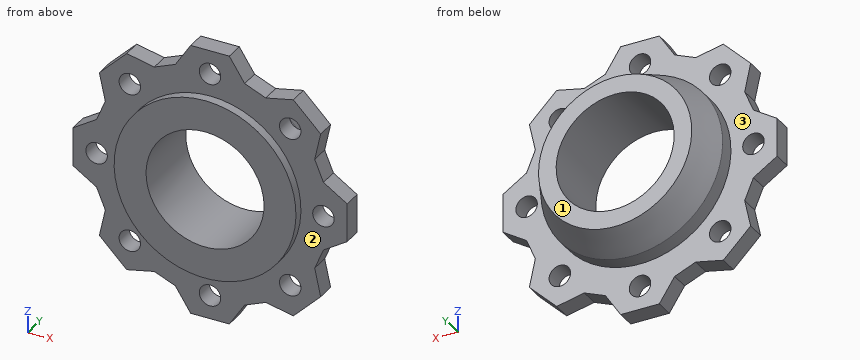
```python
from build123d import *

# Parameters (mm, degrees)
SKETCH2_R           = 3.5
SKETCH2_R_2         = 19.25
BOSS_EXTRUDE1_DEPTH = 6


with BuildPart() as part:
    # Sketch2 → Boss-Extrude1 (new body)
    with BuildSketch(Plane(origin=(0, 0, 0), x_dir=(1, 0, 0), z_dir=(0, 1, 0))):
        Polygon((27.188255737, 36.09780118), (18.172644276, 34.153257531), (11.3, 37), (6.3, 44.75), (-6.3, 44.75), (-11.3, 37), (-18.172644276, 34.153257531), (-27.188255737, 36.09780118), (-36.09780118, 27.188255737), (-34.153257531, 18.172644276), (-37, 11.3), (-44.75, 6.3), (-44.75, -6.3), (-37, -11.3), (-34.153257531, -18.172644276), (-36.09780118, -27.188255737), (-27.188255737, -36.09780118), (-18.172644276, -34.153257531), (-11.3, -37), (-6.3, -44.75), (6.3, -44.75), (11.3, -37), (18.172644276, -34.153257531), (27.188255737, -36.09780118), (36.09780118, -27.188255737), (34.153257531, -18.172644276), (37, -11.3), (44.75, -6.3), (44.75, 6.3), (37, 11.3), (34.153257531, 18.172644276), (36.09780118, 27.188255737), align=None)
        with Locations(Location((0, 37, 0), (0, 0, 270))):
            Circle(SKETCH2_R, mode=Mode.SUBTRACT)
        with Locations(Location((26.162950904, 26.162950904, 0), (0, 0, 270))):
            Circle(SKETCH2_R, mode=Mode.SUBTRACT)
        with Locations(Location((37, 0, 0), (0, 0, 270))):
            Circle(SKETCH2_R, mode=Mode.SUBTRACT)
        with Locations(Location((26.162950904, -26.162950904, 0), (0, 0, 270))):
            Circle(SKETCH2_R, mode=Mode.SUBTRACT)
        with Locations(Location((0, -37, 0), (0, 0, 270))):
            Circle(SKETCH2_R, mode=Mode.SUBTRACT)
        with Locations(Location((-26.162950904, -26.162950904, 0), (0, 0, 270))):
            Circle(SKETCH2_R, mode=Mode.SUBTRACT)
        with Locations(Location((-37, 0, 0), (0, 0, 270))):
            Circle(SKETCH2_R, mode=Mode.SUBTRACT)
        with Locations(Location((-26.162950904, 26.162950904, 0), (0, 0, 270))):
            Circle(SKETCH2_R, mode=Mode.SUBTRACT)
        with Locations(Location((0, 0, 0), (0, 0, 270))):
            Circle(SKETCH2_R_2, mode=Mode.SUBTRACT)
    extrude(amount=BOSS_EXTRUDE1_DEPTH)

    # Sketch3 → Revolve1 (revolve)
    with BuildSketch(Plane.XY, mode=Mode.PRIVATE) as revolve1_sk:
        Polygon((-19.25, 21), (-25, 21), (-29.663076582, 11), (-29.663076582, -3), (-19.25, -3), align=None)
    revolve(revolve1_sk.sketch.rotate(Axis((0, 33.758219329, 0), (0, -1, 0)), 270), axis=Axis((0, 33.758219329, 0), (0, -1, 0)))


solid = part.part
```
CAD build for the part. Positions are in the model's coordinates, mm. Face numbers are marked on the shaded views. A direction names the side the tool comes from. Round coordinates to 2 decimals unless told otherwise and drop trailing zeros. Loops run counter-clockwise (first coordinate to the right, second up) from the corner with the lowest first, then second, coordinate; pieces in that order, holes last. Notation, with made-up numbers: M 65.5,54 L 106.5,54 A11 cw 106.5,61 Z; hole C -34.5,-24 d11. An arc over 180 degrees is marked long. Return JSON: item names as keys, results as strings. Group by question number.
(1) Drop flat-ended pins along their axis: P1, Ø8, axis at x = -34.5, y = 8, coming from the -Z side; P2, Ø9, axis at x = 0, z = -37, coming from the -Y side; P3, Ø10, axis at y = 3.5, z = -12.5, coming from the -X side; P4, Ø8, axis at x = -33, y = 15, coming from the -Z side. Give the stop position or say it passes through.
(2) Saw through at A-A, the plane x = 0. List the corners of the cut face in (y, z).
(3) Wall check: probe 1 along X at (y, z) = (3.25, 0); probe 2 along X at (y, z) = (11, 0); probe 3 along Y at (x, z) = (-2, -34). Give the ranges that are in metal, low to high. Write a range as [from, to].
(4) Saw through at C-C, the plane x = -38.5. List the corners of the cut face in (y, z), and give its area (3 significant figures).
(5) Saw through at B-B, the plane z = 0. List the corners of the cut face in (x, y).
(6) Tool access for the marked faces 1, 2 and 3: list every direction of +Z, -Z, +X, -X, +Y, -Y with a clear straight run to the whole face (end or side of a thin tool).
(7) Saw through at D-D, the plane y = 16.75. List the corners of the cut face in (x, z).
Answer list:
{
 "1": {"P1": "z = -32.25", "P2": "y = 0", "P3": "x = -42.89", "P4": "through"},
 "2": {"outline": "M -3,-29.66 L 0,-29.66 L 0,-33.5 L 6,-33.5 L 6,-29.66 L 11,-29.66 L 21,-25 L 21,-19.25 L -3,-19.25 Z; M -3,19.25 L 21,19.25 L 21,25 L 11,29.66 L 6,29.66 L 6,33.5 L 0,33.5 L 0,29.66 L -3,29.66 Z; M 0,-44.75 L 6,-44.75 L 6,-40.5 L 0,-40.5 Z; M 0,40.5 L 6,40.5 L 6,44.75 L 0,44.75 Z"},
 "3": {"probe 1": "[-44.75, -40.5], [-33.5, -19.25], [19.25, 33.5], [40.5, 44.75]", "probe 2": "[-29.66, -19.25], [19.25, 29.66]", "probe 3": "[0, 6]"},
 "4": {"outline": "M 0,-10.33 L 6,-10.33 L 6,-3.16 L 0,-3.16 Z; M 0,3.16 L 6,3.16 L 6,10.33 L 0,10.33 Z", "area": "86.0 mm2"},
 "5": {"outline": "M -44.75,0 L -40.5,0 L -40.5,6 L -44.75,6 Z; M -33.5,0 L -29.66,0 L -29.66,-3 L -19.25,-3 L -19.25,21 L -25,21 L -29.66,11 L -29.66,6 L -33.5,6 Z; M 19.25,-3 L 29.66,-3 L 29.66,0 L 33.5,0 L 33.5,6 L 29.66,6 L 29.66,11 L 25,21 L 19.25,21 Z; M 40.5,0 L 44.75,0 L 44.75,6 L 40.5,6 Z"},
 "6": {"face 1": "+Z, -Z, +X, -X, +Y", "face 2": "-Y", "face 3": "+Y"},
 "7": {"outline": "C 0,0 d53.96; hole C 0,0 d38.5"}
}
